Geometry: see drawing. Coordinates: mm, zero at the bounding-box minimum. Coordinates: 2 decimals unless noted, no trailing zeros. Write each loop counter-clockwise with the first axis right and the second up, starting at its lowest first coordinate (ties: lowest second). Pieces come first, ordered by that corner, then holes. Notation, with made-up numbers: M 65.25,-6.75 L 94.25,-6.75 A26 ccw 94.25,28.25 Z; hole C -13,51.5 d9. An arc over 180 degrees is marked long. Write item = value, one per line. Start each with the question number.
1. Section query D-D (x = 102). Output: boundary loops of the cut face in (y, z) (3 decimals).
2. Line query: line 1 along Y through (x, z) = (69.85, 1.55) (3 decimals); line 2 along X through (y, z) = (106, 2.4); line 3 along X through (y, z) = (60, 2.8). Output: solid intervals per line, ascending.
3. Section query A-A (x = 69.85). Output: boundary loops of the cut face in (y, z) (3 decimals).
4. Section query C-C (y = 65). Output: boundary loops of the cut face in (x, z) (3 decimals).
5. Section query B-B (z = 2.4). Output: boundary loops of the cut face in (x, y) (3 decimals).
6. Pin query (flat end, axial travel): pin 1 Ø1 at (y, z) = (47.5, 1) entering from +X; pin 2 Ø11 at (x, y) = (69.85, 12.7) entering from +Z (3 decimals). Return the tip coordinate at first contact, or that it passes through.
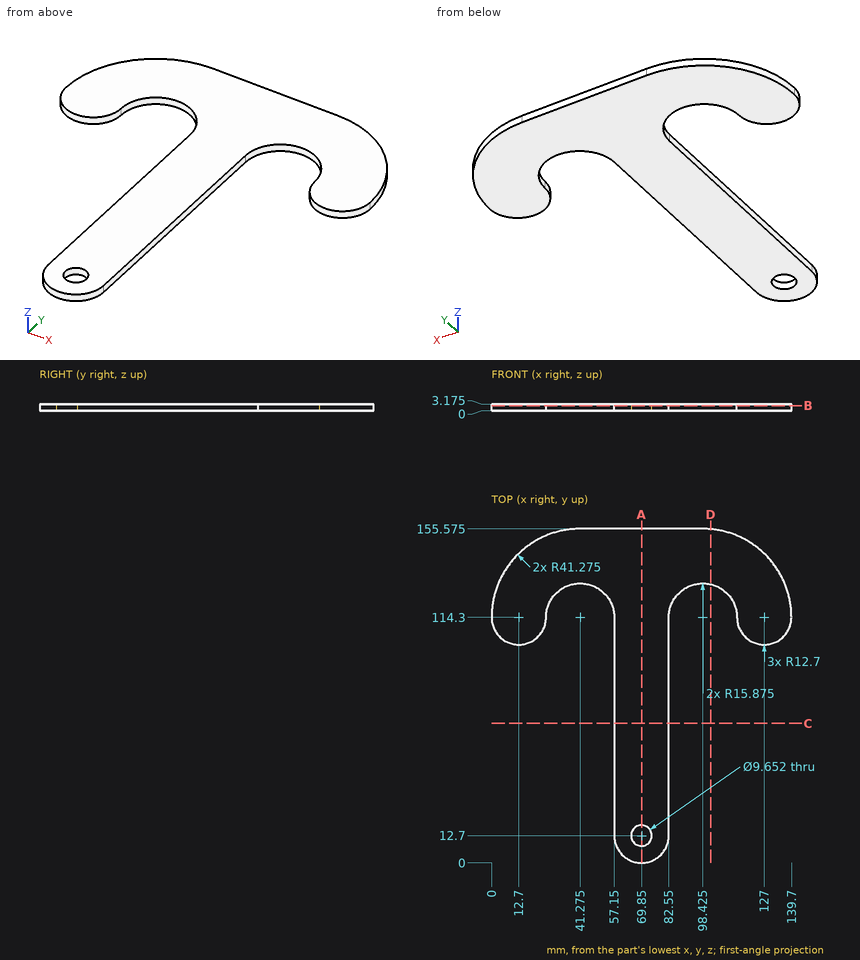
Results are:
q1.outline = M 129.767,0 L 155.42,0 L 155.42,3.175 L 129.767,3.175 Z
q2.line_1 = 0 to 7.874, 17.526 to 155.575
q2.line_2 = 3.09 to 22.31, 57.15 to 82.55, 117.39 to 136.61
q2.line_3 = 57.15 to 82.55
q3.outline = M 0,0 L 7.874,0 L 7.874,3.175 L 0,3.175 Z; M 17.526,0 L 155.575,0 L 155.575,3.175 L 17.526,3.175 Z
q4.outline = M 57.15,0 L 82.55,0 L 82.55,3.175 L 57.15,3.175 Z
q5.outline = M 0,114.3 A12.7 ccw 25.4,114.3 A15.875 cw 57.15,114.3 L 57.15,12.7 A12.7 ccw 82.55,12.7 L 82.55,114.3 A15.875 cw 114.3,114.3 A12.7 ccw 139.7,114.3 A41.275 ccw 98.425,155.575 L 41.275,155.575 A41.275 ccw Z; hole C 69.85,12.7 d9.652
q6.pin_1 = 82.55
q6.pin_2 = 3.175
